```python
from build123d import *

# Parameters (mm, degrees)
SKETCH1_R           = 5.25
BOSS_EXTRUDE1_DEPTH = 8
SKETCH2_R           = 1.5
CUT_EXTRUDE1_DEPTH  = 6
SHELL1_T            = -1.1
SKETCH3_R           = 1.5
CUT_EXTRUDE2_DEPTH  = 10.545941546
CHAMFER1_SIZE       = 1
CHAMFER2_SIZE       = 1


with BuildPart() as part:
    # Sketch1 → Boss-Extrude1 (new body)
    with BuildSketch(Plane(origin=(0, 0, 0), x_dir=(1, 0, 0), z_dir=(0, 1, 0))):
        with Locations(Location((0, 0, 0), (0, 0, 270))):
            Circle(SKETCH1_R)
    extrude(amount=BOSS_EXTRUDE1_DEPTH)

    # Sketch2 → Cut-Extrude1 (cut)
    with BuildSketch(Plane(origin=(0, 8, 0), x_dir=(1, 0, 0), z_dir=(0, 1, 0))):
        with Locations(Location((0, 0, 0), (0, 0, 270))):
            Circle(SKETCH2_R)
    extrude(amount=-CUT_EXTRUDE1_DEPTH, mode=Mode.SUBTRACT)

    # Shell1
    shell1_openings = [part.faces().sort_by_distance(p)[0] for p in [
        (0, 0, 0),
    ]]
    offset(amount=SHELL1_T, openings=shell1_openings, kind=Kind.INTERSECTION)

    # Sketch3 → Cut-Extrude2 (cut, through all)
    with BuildSketch(Plane(origin=(0, 2, 0), x_dir=(1, 0, 0), z_dir=(0, 1, 0))):
        with Locations(Location((0, 0, 0), (0, 0, 270))):
            Circle(SKETCH3_R)
    extrude(amount=-CUT_EXTRUDE2_DEPTH, mode=Mode.SUBTRACT)

    # Chamfer1
    chamfer1_edges = [part.edges().sort_by_distance(p)[0] for p in [
        (0, 8, -5.25),
    ]]
    chamfer(chamfer1_edges, length=CHAMFER1_SIZE)

    # Chamfer2
    chamfer2_edges = [part.edges().sort_by_distance(p)[0] for p in [
        (0, 8, -1.5),
    ]]
    chamfer(chamfer2_edges, length=CHAMFER2_SIZE)


solid = part.part
```
Design review of the part built by this model. Coordinates are the model's own, in mm. A direction names the side the tool comes from. Round coordinates to 2 decimals unless told otherwise and drop trailing zeros. Order: outer loops, then holes, each group sorted by start corner. A loop starts at its lowest first (then second) coordinate and runs counter-clockwise, first axis right, second up. Notation, with made-up numbers: (34.25, 1) - (81.25, 1) arc R30 ccw to (81.25, 27) - close; hole circle Ø6 at (38.5, 58). An arc over 180 degrees is marked (long way). One line per question, with ' | ' between items.
Item 1: Take a section at B-B, the plane y = 3.25. Write out the cut boundary in (x, z), then the cut area to 3 significant figures.
Checks:
outline: circle Ø10.5 at (0, 0); circle Ø5.2 at (0, 0); hole circle Ø8.3 at (0, 0); hole circle Ø3 at (0, 0) | area: 46.7 mm²
Item 2: Draft analysis for pull direction Z (two halves, no side actions). For faces 3 (the face through (1.6, 3.5, 5)), 4 (the face through (0.78, 3.94, 2.48)), 5 (the face through (2, 0, 4)), state which applies: +Z half, -Z half, draft (parallel to the pull), parting line (faces both ways), or undercut.
Checks:
face 3: parting line | face 4: undercut | face 5: draft
Item 3: Take a section at C-C, the plane z = 0. Write out the cut boundary in (x, y).
Checks:
outline: (-5.25, 0) - (-4.15, 0) - (-4.15, 6.9) - (-2.6, 6.9) - (-2.6, 0.9) - (-1.5, 0.9) - (-1.5, 7) - (-2.5, 8) - (-4.25, 8) - (-5.25, 7) - close; (1.5, 0.9) - (2.6, 0.9) - (2.6, 6.9) - (4.15, 6.9) - (4.15, 0) - (5.25, 0) - (5.25, 7) - (4.25, 8) - (2.5, 8) - (1.5, 7) - close
Item 4: For P1, Ø4, axis at x = 0, z = 0, coming from the -Y side; P2, Ø2, axis at x = 3.5, y = 6.5, coming from the -Z side; P3, Ø1.5, axis at y = 1, z = 2, coming from the +X side, all flat-tipped, find the tip position at first contact; note any pin that passes through.
Checks:
P1: y = 0.9 | P2: z = -4.62 | P3: x = 5.1
Item 5: Take a section at A-A, the plane x = 0. Write out the cut boundary in (y, z).
Checks:
outline: (0, -5.25) - (7, -5.25) - (8, -4.25) - (8, -2.5) - (7, -1.5) - (0.9, -1.5) - (0.9, -2.6) - (6.9, -2.6) - (6.9, -4.15) - (0, -4.15) - close; (0, 4.15) - (6.9, 4.15) - (6.9, 2.6) - (0.9, 2.6) - (0.9, 1.5) - (7, 1.5) - (8, 2.5) - (8, 4.25) - (7, 5.25) - (0, 5.25) - close
Item 6: Take a section at D-D, the plane y = 0.5. Write out the cut boundary in (x, z), then the cut area to 3 significant figures.
Checks:
outline: circle Ø10.5 at (0, 0); hole circle Ø8.3 at (0, 0) | area: 32.5 mm²
Item 7: Machinability: for faces 1 (the face through (-2, 0.9, 0)), 2 (the face through (-2, 8, 2)), which of the approach directions +Z, -Z, +X, -X, +Y, -Y give a long, thin tool a straight path to every point of the face, cutting with its end or side? Answer none if there is none.
Checks:
face 1: -Y | face 2: +Z, -Z, +X, -X, +Y
Item 8: Wall thickness on line 1 (X direction, y = 4, z = 0); line 2 (Z direction, x = -0.5, y = 6.5); line 3 (Z direction, x = -0.25, y = 6.75): over which ranges is each line inside the solid? List them lowest first. Write a range as [from, to].
Checks:
line 1: [-5.25, -4.15], [-2.6, -1.5], [1.5, 2.6], [4.15, 5.25] | line 2: [-5.23, -4.12], [-2.55, -1.41], [1.41, 2.55], [4.12, 5.23] | line 3: [-5.24, -4.14], [-2.59, -1.48], [1.48, 2.59], [4.14, 5.24]
